from build123d import *

# Parameters (mm, degrees)
SKETCH1_W                          = 18
SKETCH1_H                          = 19
BOSS_EXTRUDE1_DEPTH                = 2
SKETCH2_W                          = 29
SKETCH2_H                          = 4
BOSS_EXTRUDE2_DEPTH                = 30
M3_CLEARANCE_HOLE1_D               = 3.2
TAPPED_HOLE_FOR_M4X0_7_HELICOIL1_D = 4.2


with BuildPart() as part:
    # Sketch1 → Boss-Extrude1 (new, symmetric)
    with BuildSketch(Plane.XY):
        Rectangle(SKETCH1_W, SKETCH1_H)
    extrude(amount=BOSS_EXTRUDE1_DEPTH, both=True)

    # Sketch2 → Boss-Extrude2 (add)
    with BuildSketch(Plane(origin=(0, 0, 2), x_dir=(-1, 0, 0), z_dir=(0, 0, -1))):
        with Locations((5.5, -7.5)):
            Rectangle(SKETCH2_W, SKETCH2_H)
    extrude(amount=BOSS_EXTRUDE2_DEPTH)

    # M3 Clearance Hole1 (through all)
    with Locations(Plane.XY.offset(2)):
        with Locations((-5.715, 4.5028), (5.715, 4.5028)):
            Hole(M3_CLEARANCE_HOLE1_D / 2)

    # Tapped Hole for M4x0.7 Helicoil1 (through all)
    with Locations(Plane(origin=(0, -9.5, 0), x_dir=(-1, 0, 0), z_dir=(0, -1, 0))):
        with Locations((14.9858, 17.875)):
            Hole(TAPPED_HOLE_FOR_M4X0_7_HELICOIL1_D / 2)


solid = part.part
Design review of the part built by this model. Coordinates are the model's own, in mm. A direction names the side the tool comes from. Coordinates: 2 decimals unless noted, no trailing zeros. Order: outer loops, then holes, each group sorted by start corner. A loop starts at its lowest first (then second) coordinate and runs counter-clockwise, first axis right, second up. Notation, with made-up numbers: (6.5, 53) -> (29.5, 53) arc R14 cw to (29.5, 67) -> close; hole circle Ø1 at (31, 69.25). An arc over 180 degrees is marked (long way). One line per item, written item: value.
1) Machinability: for faces 1 (the face through (-12.983, -7.472, -18.506)), 2 (the face through (-9, 2, 0)), 3 (the face through (0, 2, -2)), which of the approach directions +Z, -Z, +X, -X, +Y, -Y give a long, thin tool a straight path to every point of the face, cutting with its end or side? Answer none if there is none.
Output values:
face 1: +Y, -Y
face 2: +Z, -Z, -X, +Y
face 3: -Z, +X, -X, +Y
2) We need section C-C, the plane z = -16.5. Give the boundary of the cut face in (x, y).
Output values:
outline: (-20, -9.5) -> (-16.57, -9.5) -> (-16.57, -5.5) -> (-20, -5.5) -> close; (-13.4, -9.5) -> (9, -9.5) -> (9, -5.5) -> (-13.4, -5.5) -> close
3) Draft analysis for pull direction X (two halves, no side actions). For faces 4 (the face through (9, -6, -10)), 5 (the face through (6.894, 5.584, -0.028)), 6 (the face through (-2, 0, 2)), state which applies: +X half, -X half, draft (parallel to the pull), parting line (faces both ways), or undercut.
Output values:
face 4: +X half
face 5: undercut
face 6: draft
4) To check wall thickness, follow probe 1 along Y at (x, z) = (-11.25, -17.25); probe 2 along X at (y, z) = (7, 0.5); probe 3 along Z at (x, y) = (3, 1.5). State the ranges of each line that lie inside material, in increasing order. Write a range as [from, to].
Output values:
probe 1: y = [-9.5, -5.5]
probe 2: x = [-9, 9]
probe 3: z = [-2, 2]
5) Clearance check with flat-ended pins moving along their axes: P1, Ø14.5, axis at x = -11.5, z = -17.5, coming from the +Y side; P2, Ø3, axis at y = -1, z = 0, coming from the -X side; P3, Ø7.5, axis at x = -2, y = 5, coming from the -Z side. State where each tip first meets the part, or that it passes through.
Output values:
P1: stops at y = -5.5
P2: stops at x = -9
P3: stops at z = -2
6) We need section D-D, the plane z = 0.25. Give the boundary of the cut face in (x, y) (3 decimals), then the cut area to 3 significant figures.
Output values:
outline: (-20, -9.5) -> (9, -9.5) -> (9, 9.5) -> (-9, 9.5) -> (-9, -5.5) -> (-20, -5.5) -> close; hole circle Ø3.2 at (-5.715, 4.503); hole circle Ø3.2 at (5.715, 4.503)
area: 370 mm2
7) We need section B-B, the plane y = 5.5. Give the boundary of the cut face in (x, z).
Output values:
outline: (-9, -2) -> (-6.97, -2) -> (-6.97, 2) -> (-9, 2) -> close; (-4.46, -2) -> (4.46, -2) -> (4.46, 2) -> (-4.46, 2) -> close; (6.97, -2) -> (9, -2) -> (9, 2) -> (6.97, 2) -> close
8) We need section A-A, the plane x = 6.75. Give the boundary of the cut face in (y, z), then the cut area to 3 significant figures.
Output values:
outline: (-9.5, -28) -> (-5.5, -28) -> (-5.5, -2) -> (3.28, -2) -> (3.28, 2) -> (-9.5, 2) -> close; (5.72, -2) -> (9.5, -2) -> (9.5, 2) -> (5.72, 2) -> close
area: 170 mm2
